```python
from build123d import *

# Parameters (mm, degrees)
SALIENTE_EXTRUIR1_DEPTH = 50
CROQUIS2_R              = 5.032013792
CORTAR_EXTRUIR1_DEPTH   = 10


with BuildPart() as part:
    # Croquis1 → Saliente-Extruir1 (new body)
    with BuildSketch(Plane.XY):
        with BuildLine():
            Line((0, 0), (0, -25))
            ThreePointArc((0, -25), (7.725424859, -23.776412907), (14.694631307, -20.225424859))
            Line((14.694631307, -20.225424859), (0, 0))
        make_face()
    extrude(amount=SALIENTE_EXTRUIR1_DEPTH)

    # Croquis2 → Cortar-Extruir1 (cut)
    with BuildSketch(Plane(origin=(0, 0, 0), x_dir=(-1, 0, 0), z_dir=(0, 0, -1))):
        with Locations((-5.939812616, -18.149032461)):
            Circle(CROQUIS2_R)
    extrude(amount=-CORTAR_EXTRUIR1_DEPTH, mode=Mode.SUBTRACT)


solid = part.part
```
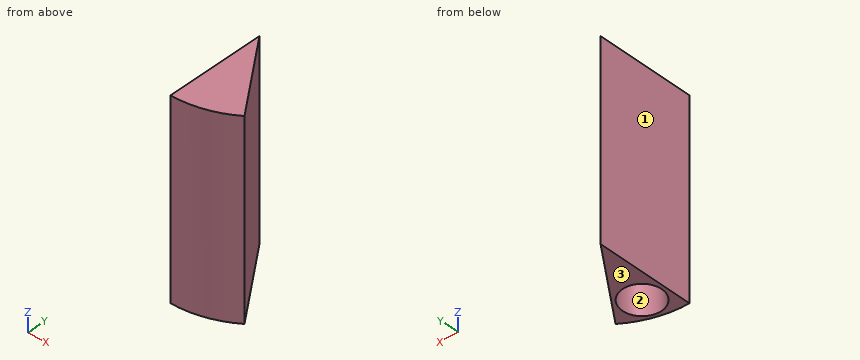
Geometry check sheet. Reference: the model listing, model coordinates, mm. Face numbers are marked on the shaded views. Coordinates: 2 decimals unless noted, no trailing zeros. Order: outer loops, then holes, each group sorted by start corner. A loop starts at its lowest first (then second) coordinate and runs counter-clockwise, first axis right, second up. Notation, with made-up numbers: (37.5, 26.25) - (68.5, 26.25) arc R17 cw to (68.5, 41.25) - close; hole circle Ø2 at (-14, 40). An arc over 180 degrees is marked (long way). Answer in a Markdown table with one row per item. Add a question column.
1. Section check A-A (y = -22). Enter the section's corners in (x, z), plus the area to 3 significant figures.
2. Gauge pin test, flat ends, axial feed: pin 1 Ø8 at (x, y) = (6.5, -17.5) entering from -Z; pin 2 Ø1.5 at (y, z) = (-12.5, 15.5) entering from +X; pin 3 Ø1.5 at (y, z) = (-4, 20.5) entering from +X. Record the tip position at first contact, or that the pin passes through.
3. Material ranges on L1, parallel to Z at x = 7.5, y = -21.25; L2, parallel to Y at x = 2, z = 14; L3, parallel to X at y = -16, z = 32, recorded low to high. Write a range as [from, to].
4. Draft check along X on the marked faces 1, 2 and 3. Enter one of: +X half, -X half, draft (parallel to the pull), parting line (faces both ways), or undercut.
5. Section check C-C (z = 9). Enter the section's corners in (x, y).
6. Section check D-D (y = -8.5). Enter the section's corners in (x, z).
7. Section check B-B (x = 8.25). Enter the section's corners in (y, z), plus the area to 3 significant figures.
Data:
| question | item | result |
|---|---|---|
| 1 | outline | (0, 0) - (2.7, 0) - (2.7, 10) - (9.18, 10) - (9.18, 0) - (11.87, 0) - (11.87, 50) - (0, 50) - close |
| 1 | area | 529 mm² |
| 2 | pin 1 | stops at z = 10 |
| 2 | pin 2 | stops at x = 9.63 |
| 2 | pin 3 | stops at x = 3.45 |
| 3 | L1 | z = [10, 50] |
| 3 | L2 | y = [-24.92, -2.75] |
| 3 | L3 | x = [0, 11.62] |
| 4 | face 1 | -X half |
| 4 | face 2 | undercut |
| 4 | face 3 | draft |
| 5 | outline | (0, -25) arc R25 ccw to (14.69, -20.23) - (0, 0) - close; hole circle Ø10.06 at (5.94, -18.15) |
| 6 | outline | (0, 0) - (6.18, 0) - (6.18, 50) - (0, 50) - close |
| 7 | outline | (-23.6, 0) - (-22.62, 0) - (-22.62, 10) - (-13.68, 10) - (-13.68, 0) - (-11.36, 0) - (-11.36, 50) - (-23.6, 50) - close |
| 7 | area | 523 mm² |
